Check sheet for the modelled part. Datum: model origin and axes. Units: mm. A direction names the side the tool comes from. Round coordinates to 2 decimals unless told otherwise and drop trailing zeros. Answer as a JSON object with one key per item and string values. Group by question number.
Item 1: Thickness scan on line 1 (X direction, y = 43.75, z = 12.5) (3 decimals); line 2 (Y direction, x = -69.5, z = 10.5) (3 decimals); line 3 (Y direction, x = -12, z = 8). Record the ranges inside material, lowest first.
Item 2: Set-up check for faces 1 (the flat face through (-101.359, 24.475, 18.916)), 2 (the cylindrical face through (-71.86, 6.99, 13.66)): record each of +Z, -Z, +X, -X, +Y, -Y from which the full face is reachable in a straight line by a thin tool's end or side.
Item 3: Gauge pin test, flat end, axial feed: P1, Ø6.5, axis at x = -69.5, y = 43.75, coming from the +Z side. Record the tip position at first contact, or that the pin passes through.
Item 4: Release check for a two-part mould opening along Y. For faces 3 (the flat face through (-41.861, -11.359, 18.916)), 4 (the cylindrical face through (-71.86, 44.49, 13.66)), 5 (the flat face through (-42, 26, -3.975)) record: pulls with the +Y half, pulls with the -Y half, needs draft (parallel to the pull), parting line crosses it, or undercut.
```python
from build123d import *

# Parameters (mm, degrees)
SKETCH1_W                   = 82
SKETCH1_H                   = 50
BOSS_EXTRUDE4_DEPTH         = 16
M4_TAPPED_HOLE1_D           = 3.3
M4_TAPPED_HOLE1_DEPTH       = 8
M4_TAPPED_HOLE1_CSINK_D     = 4.05
M4_TAPPED_HOLE1_CSINK_ANGLE = 90
M4_TAPPED_HOLE1_TIP         = 0.991420021
CHAMFER1_SIZE               = 1.5
SCALE1_SCALE                = 1.5


with BuildPart() as part:
    # Sketch1 → Boss-Extrude4 (new body)
    with BuildSketch(Plane.XY):
        with Locations((-41, 25)):
            Rectangle(SKETCH1_W, SKETCH1_H)
    extrude(amount=BOSS_EXTRUDE4_DEPTH)

    # M4 Tapped Hole1
    with Locations(Plane.XY.offset(16)):
        with Locations((-60, 37.5), (-60, 12.5), (-22, 12.5), (-22, 37.5)):
            CounterSinkHole(M4_TAPPED_HOLE1_D / 2, M4_TAPPED_HOLE1_CSINK_D / 2, depth=M4_TAPPED_HOLE1_DEPTH, counter_sink_angle=M4_TAPPED_HOLE1_CSINK_ANGLE)
            with Locations((0, 0, -(M4_TAPPED_HOLE1_DEPTH + M4_TAPPED_HOLE1_TIP / 2))):  # 118° drill point
                Cone(0, M4_TAPPED_HOLE1_D / 2, M4_TAPPED_HOLE1_TIP, mode=Mode.SUBTRACT)

    # Chamfer1
    chamfer1_edges = [part.edges().sort_by_distance(p)[0] for p in [
        (-82, 25, 16),
        (-41, 0, 16),
        (0, 25, 16),
        (-41, 50, 16),
    ]]
    chamfer(chamfer1_edges, length=CHAMFER1_SIZE)


with BuildPart() as part_1:
    # Scale1: scaled about (-41, 25, 7.949093999)
    add(part.part.scale(SCALE1_SCALE).moved(Location((20.5, -12.5, -3.974546999))))


solid = part_1.part
```
Completed:
{
 "1": {"line 1": "-102.5 to -71.975, -67.025 to -14.975, -10.025 to 20.5", "line 2": "-12.5 to 3.775, 8.725 to 41.275, 46.225 to 62.5", "line 3": "-12.5 to 3.87, 8.63 to 41.37, 46.13 to 62.5"},
 "2": {"face 1": "+Z, -X, +Y, -Y", "face 2": "+Z"},
 "3": {"P1": "z = 20.03"},
 "4": {"face 3": "pulls with the -Y half", "face 4": "undercut", "face 5": "needs draft"}
}
